```python
from build123d import *

# Parameters (mm, degrees)
SKETCH1_R           = 35.5
BOSS_EXTRUDE1_DEPTH = 2.5
SKETCH2_R           = 26
BOSS_EXTRUDE2_DEPTH = 1
SKETCH3_R           = 25
BOSS_EXTRUDE3_DEPTH = 19
CHAMFER1_SIZE       = 1
SKETCH4_R           = 12
CUT_EXTRUDE1_DEPTH  = 57.084757288
SKETCH5_R           = 7.5
CUT_EXTRUDE2_DEPTH  = 57.084757332
FILLET1_R           = 1
SKETCH6_R           = 30.018937713
SKETCH6_R_2         = 20
CUT_EXTRUDE3_DEPTH  = 12
CHAMFER2_SIZE       = 2.5
SKETCH7_R           = 1.75
CUT_EXTRUDE4_DEPTH  = 57.084757332
CUT_EXTRUDE5_DEPTH  = 3
SKETCH9_R           = 1.75
CUT_EXTRUDE6_DEPTH  = 55.041650641
CHAMFER3_SIZE       = 2


# Some blends are built 0.0001 mm under size
with BuildPart() as part:
    # Sketch1 → Boss-Extrude1 (new, symmetric)
    with BuildSketch(Plane(origin=(0, 0, 0), x_dir=(1, 0, 0), z_dir=(0, 1, 0))):
        with Locations(Location((0, 0, 0), (0, 0, 270))):
            Circle(SKETCH1_R)
    extrude(amount=BOSS_EXTRUDE1_DEPTH, both=True)

    # Sketch2 → Boss-Extrude2 (add)
    with BuildSketch(Plane(origin=(0, 2.5, 0), x_dir=(1, 0, 0), z_dir=(0, 1, 0))):
        with Locations(Location((0, 0, 0), (0, 0, 270))):
            Circle(SKETCH2_R)
    extrude(amount=BOSS_EXTRUDE2_DEPTH)

    # Sketch3 → Boss-Extrude3 (add)
    with BuildSketch(Plane(origin=(0, 3.5, 0), x_dir=(1, 0, 0), z_dir=(0, 1, 0))):
        with Locations(Location((0, 0, 0), (0, 0, 270))):
            Circle(SKETCH3_R)
    extrude(amount=BOSS_EXTRUDE3_DEPTH)

    # Chamfer1
    chamfer1_edges = [part.edges().sort_by_distance(p)[0] for p in [
        (0, 2.5, -26),
    ]]
    chamfer(chamfer1_edges, length=CHAMFER1_SIZE - 0.0001)  # a hair under: the kernel refuses the full size

    # Sketch4 → Cut-Extrude1 (cut, through all)
    with BuildSketch(Plane(origin=(0, 22.5, 0), x_dir=(1, 0, 0), z_dir=(0, 1, 0))):
        with Locations(Location((0, 15.5, 0), (0, 0, 270))):
            Circle(SKETCH4_R)
        with Locations(Location((13.423393759, -7.75, 0), (0, 0, 270))):
            Circle(SKETCH4_R)
        with Locations(Location((-13.423393759, -7.75, 0), (0, 0, 270))):
            Circle(SKETCH4_R)
    extrude(amount=-CUT_EXTRUDE1_DEPTH, mode=Mode.SUBTRACT)

    # Sketch5 → Cut-Extrude2 (cut, through all)
    with BuildSketch(Plane(origin=(0, 22.5, 0), x_dir=(1, 0, 0), z_dir=(0, 1, 0))):
        Circle(SKETCH5_R)
    extrude(amount=-CUT_EXTRUDE2_DEPTH, mode=Mode.SUBTRACT)

    # Fillet1
    fillet1_edges = [part.edges().sort_by_distance(p)[0] for p in [
        (-15.575022283, 13, 19.555528141),
        (-24.723095296, 13, 3.710600891),
        (24.723095296, 13, 3.710600891),
        (15.575022283, 13, 19.555528141),
        (-9.148073013, 13, -23.266129032),
        (9.148073013, 13, -23.266129032),
    ]]
    fillet(fillet1_edges, radius=FILLET1_R)

    # Sketch6 → Cut-Extrude3 (cut)
    with BuildSketch(Plane(origin=(0, 22.5, 0), x_dir=(1, 0, 0), z_dir=(0, 1, 0))):
        Circle(SKETCH6_R)
        Circle(SKETCH6_R_2, mode=Mode.SUBTRACT)
    extrude(amount=-CUT_EXTRUDE3_DEPTH, mode=Mode.SUBTRACT)

    # Chamfer2
    chamfer2_edges = [part.edges().sort_by_distance(p)[0] for p in [
        (17.320508076, 10.5, -10),
        (-17.320508076, 10.5, -10),
        (0, 10.5, 20),
    ]]
    chamfer(chamfer2_edges, length=CHAMFER2_SIZE)

    # Sketch7 → Cut-Extrude4 (cut, through all)
    with BuildSketch(Plane(origin=(0, 22.5, 0), x_dir=(1, 0, 0), z_dir=(0, 1, 0))):
        with Locations(Location((0, -15, 0), (0, 0, 270))):
            Circle(SKETCH7_R)
        with Locations(Location((-12.990381057, 7.5, 0), (0, 0, 270))):
            Circle(SKETCH7_R)
        with Locations(Location((12.990381057, 7.5, 0), (0, 0, 270))):
            Circle(SKETCH7_R)
    extrude(amount=-CUT_EXTRUDE4_DEPTH, mode=Mode.SUBTRACT)

    # Sketch8 → Cut-Extrude5 (cut)
    with BuildSketch(Plane.XZ.offset(2.5)):
        Polygon((18.879353803, -9), (17.233905535, -6.15), (13.943009001, -6.15), (12.297560734, -9), (13.943009001, -11.85), (17.233905535, -11.85), align=None)
        Polygon((-1.645448267, 17.85), (-3.290896534, 15), (-1.645448267, 12.15), (1.645448267, 12.15), (3.290896534, 15), (1.645448267, 17.85), align=None)
        Polygon((-14.635829324, -13.35), (-11.34493279, -13.35), (-9.699484522, -10.5), (-11.34493279, -7.65), (-14.635829324, -7.65), (-16.281277591, -10.5), align=None)
    extrude(amount=-CUT_EXTRUDE5_DEPTH, mode=Mode.SUBTRACT)

    # Sketch9 → Cut-Extrude6 (cut, through all)
    with BuildSketch(Plane(origin=(0, 2.5, 0), x_dir=(1, 0, 0), z_dir=(0, 1, 0))):
        with Locations(Location((-4.453539231, 31.6885782, 0), (0, 0, 270))):
            Circle(SKETCH9_R)
        with Locations(Location((29.669883346, -11.987410989, 0), (0, 0, 270))):
            Circle(SKETCH9_R)
        with Locations(Location((-25.216344115, -19.70116721, 0), (0, 0, 270))):
            Circle(SKETCH9_R)
    extrude(amount=-CUT_EXTRUDE6_DEPTH, mode=Mode.SUBTRACT)

    # Chamfer3
    # the kernel refuses this chamfer: 2 mm, written as the material it takes off along each edge
    with BuildSketch(Plane(origin=(-4.453539231, 2.5, -31.6885782), x_dir=(0, 0, 1), z_dir=(-1, 0, 0))) as chamfer3_piece_1:
        Polygon((1.75 + CHAMFER3_SIZE, 0), (1.75, -CHAMFER3_SIZE), (1.75, 0), align=None)
    revolve(axis=Axis((-4.453539231, 2.5, -31.6885782), (0, 1, 0)), mode=Mode.SUBTRACT)
    with BuildSketch(Plane(origin=(29.669883346, 2.5, 11.987410989), x_dir=(0, 0, 1), z_dir=(-1, 0, 0))) as chamfer3_piece_2:
        Polygon((1.75 + CHAMFER3_SIZE, 0), (1.75, -CHAMFER3_SIZE), (1.75, 0), align=None)
    revolve(axis=Axis((29.669883346, 2.5, 11.987410989), (0, 1, 0)), mode=Mode.SUBTRACT)
    with BuildSketch(Plane(origin=(-25.216344115, 2.5, 19.70116721), x_dir=(0, 0, 1), z_dir=(-1, 0, 0))) as chamfer3_piece_3:
        Polygon((1.75 + CHAMFER3_SIZE, 0), (1.75, -CHAMFER3_SIZE), (1.75, 0), align=None)
    revolve(axis=Axis((-25.216344115, 2.5, 19.70116721), (0, 1, 0)), mode=Mode.SUBTRACT)


solid = part.part
```
Could you check a few things on this model? Use its own coordinates, in mm. A direction names the side the tool comes from. Coordinates: 2 decimals unless noted, no trailing zeros. Loops run counter-clockwise (first coordinate to the right, second up) from the corner with the lowest first, then second, coordinate; pieces in that order, holes last. Notation, with made-up numbers: M 85,18.5 L 126,18.5 A23 ccw 126,27.5 Z; hole C 29,-40 d8. An arc over 180 degrees is marked long. Put each result on its own line as item: value. Start each with the question number.
(1) For faces 4 (the face through (17.38, 17.82, -9.9)), 5 (the face through (-17.264, 17.816, -10.098)), 6 (the face through (6.505, 10.175, -3.733)), 7 (the face through (-2.48, -1.021, 13.595)), 8 (the face through (0, 7, 25)), which set-ups out of +Z, -Z, +X, -X, +Y, -Y let a thin tool reach every point of the face, with its end or its side?
(2) Suppose I cut it at B-B on y = 6.5. Count the separate pieces of the cut face and the enclosed holes in it, then the cut area to 3 significant figures.
(3) Thinking about a two-plate mould opening in Z: for faces 1 (the face through (-6.485, 10.175, -3.767)), 2 (the face through (-14.2, 22.5, -9.3)), 3 (the face through (-0.3, 3.3, 26.2)), which applies, pulls with the +Z half, pulls with the -Z half, needs draft (parallel to the pull), parting line crosses it, or undercut?
(4) Will these pins go through, and if not, where does the flat tip stop? P1, Ø1, axis at y = 18.5, z = 13.5, coming from the -X side; P2, Ø1, axis at x = -17.5, y = 9.5, coming from the +Z side; P3, Ø4.5, axis at x = -12.99, z = -7.5, coming from the +Y side; P4, Ø1, axis at x = -10, y = 20, coming from the -Z side.
(5) Suppose I cut it at A-A on y = 19.25. Please give me the cut outline in (x, z).
(6) I need wall thicknesses on line 1 (X direction, y = 5, z = -7); line 2 (X direction, y = -1.25, z = 8.5); line 3 (X direction, y = 16, z = -3). Which ranges of each line are inside material? Lowest first, please. Write a range as from..to.
Solutions:
1. face 4: -Z, +X, +Y
1. face 5: -Z, -X, +Y
1. face 6: +Y, -Y
1. face 7: -Y
1. face 8: +Z, +Y
2. separate pieces: 3
2. enclosed holes: 3
2. area: 579 mm2
3. face 1: undercut
3. face 2: needs draft
3. face 3: pulls with the +Z half
4. P1: stops at x = -3.18
4. P2: stops at z = -3.34
4. P3: stops at y = 22.5
4. P4: stops at z = -9.69
5. outline: M -19.86,-2.38 A20 ccw -11.99,-16.01 A12 cw -5.66,-4.92 A7.5 cw -7.09,-2.44 A12 cw Z; M -7.87,18.39 A12 cw -1.43,7.36 A7.5 cw 1.43,7.36 A12 cw 7.87,18.39 A20 ccw Z; M 5.66,-4.92 A12 cw 11.99,-16.01 A20 ccw 19.86,-2.38 A12 cw 7.09,-2.44 A7.5 cw Z; hole C -12.99,-7.5 d3.5; hole C 0,15 d3.5; hole C 12.99,-7.5 d3.5
6. line 1: x = -24..-14.67, -11.31..-8.47, 8.47..11.31, 14.67..24
6. line 2: x = -34.47..-25.4, -1.45..1.45, 25.4..34.47
6. line 3: x = -19.77..-18.76, -8.09..-6.87, 6.87..8.09, 18.76..19.77
